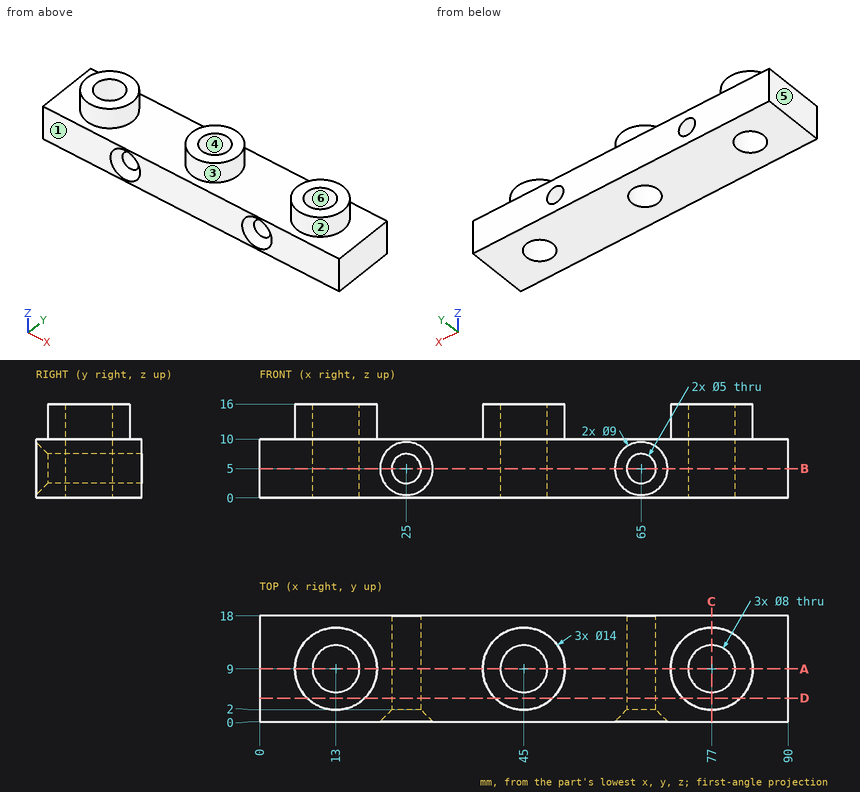
Source: three-view drawing plus pictorial views. Frame: mm from the lowest corner of the part. A direction names the side the tool comes from. Coordinates: 2 decimals unless noted, no trailing zeros. Loops run counter-clockwise (first coordinate to the right, second up) from the corner with the lowest first, then second, coordinate; pieces in that order, holes last. Notation, with made-up numbers: (7, 62) - (13, 62) arc R19 cw to (13, 76) - close; hole circle Ø10 at (25.5, 74). An arc over 180 degrees is marked (long way). One line per item, written item: value. Start each with the question number.
1. Section B-B (z = 5). Return the cut outline in (x, y), and give its area (3 significant figures).
2. Set-up query: the marked faces 1 and 2. Return all of +Z, -Z, +X, -X, +Y, -Y with unobstructed straight access to the full face (end or side cutting, diameter ignored); none if empty.
3. Mould query, pull axis Y, two halves, no side actions, for the marked faces 3, 4, 5 and 6. Classes: pulls with the +Y half, pulls with the -Y half, needs draft (parallel to the pull), parting line crosses it, or undercut.
4. Ray query, L1, parallel to Y at x = 77, z = 12.75; L2, parallel to Z at x = 25, y = 10; L3, parallel to Y at x = 45, z = 4.5. Return the intervals inside material, ascending.
5. Section C-C (x = 77). Return the cut outline in (y, z), and give its area (3 significant figures).
6. Section A-A (y = 9). State how many separate pieces and enclosed holes the cut face has, and give its area (3 significant figures).
7. Section D-D (y = 4). Return the cut outline in (x, z).
8. Contact query for a flat-ended pin moving along its axis: P1, Ø3, axis at x = 59, y = 15.5, coming from the +Z side. Output: stop coordinate, or through.
Verdict:
1. outline: (0, 0) - (20.5, 0) - (22.5, 2) - (22.5, 18) - (0, 18) - close; (27.5, 2) - (29.5, 0) - (60.5, 0) - (62.5, 2) - (62.5, 18) - (27.5, 18) - close; (67.5, 2) - (69.5, 0) - (90, 0) - (90, 18) - (67.5, 18) - close; hole circle Ø8 at (13, 9); hole circle Ø8 at (45, 9); hole circle Ø8 at (77, 9)
1. area: 1,280 mm2
2. face 1: +Z, -Z, +X, -X, -Y
2. face 2: +Z
3. face 3: parting line crosses it
3. face 4: undercut
3. face 5: needs draft
3. face 6: undercut
4. L1: y = 2 to 5, 13 to 16
4. L2: z = 0 to 2.5, 7.5 to 10
4. L3: y = 0 to 5, 13 to 18
5. outline: (0, 0) - (5, 0) - (5, 16) - (2, 16) - (2, 10) - (0, 10) - close; (13, 0) - (18, 0) - (18, 10) - (16, 10) - (16, 16) - (13, 16) - close
5. area: 136 mm2
6. separate pieces: 4
6. enclosed holes: 2
6. area: 729 mm2
7. outline: (0, 0) - (90, 0) - (90, 10) - (81.9, 10) - (81.9, 16) - (72.1, 16) - (72.1, 10) - (49.9, 10) - (49.9, 16) - (40.1, 16) - (40.1, 10) - (17.9, 10) - (17.9, 16) - (8.1, 16) - (8.1, 10) - (0, 10) - close; hole circle Ø5 at (25, 5); hole circle Ø5 at (65, 5)
8. P1: stops at z = 10
